```python
from build123d import *

# Parameters (mm, degrees)
CUT_EXTRUDE1_DEPTH             = 115.3
CUT_EXTRUDE1_DEPTH_BACK        = 115.3
BOSS_EXTRUDE1_DEPTH            = 142.875
BOSS_EXTRUDE2_DEPTH            = 22.225
CUT_EXTRUDE2_REACH             = 119.475
CUT_EXTRUDE2_DIRECTION_2_REACH = 119.475


with BuildPart() as part:
    # Sketch1 → Revolve1 (revolve)
    with BuildSketch(Plane(origin=(0, 0, 0), x_dir=(0, 0, -1), z_dir=(1, 0, 0))):
        with BuildLine():
            Line((-76.2, -52.3875), (-117.475, -52.3875))
            Line((-117.475, -52.3875), (-117.475, -114.3))
            Line((-117.475, -114.3), (-95.25, -114.3))
            Line((-95.25, -114.3), (-95.25, -68.2625))
            Line((-95.25, -68.2625), (-76.2, -68.2625))
            Line((-76.2, -68.2625), (-71.4375, -73.025))
            Line((-71.4375, -73.025), (-41.936651857, -73.025))
            ThreePointArc((-41.936651857, -73.025), (-43.560758987, -70.75739219), (-44.836334568, -68.276933343))
            ThreePointArc((-44.836334568, -68.276933343), (-47.073606935, -62.750045829), (-49.120888044, -57.15))
            Line((-49.120888044, -57.15), (-71.4375, -57.15))
            Line((-71.4375, -57.15), (-76.2, -52.3875))
        make_face()
        with BuildLine():
            ThreePointArc((0, -73.025), (15.290494263, -71.406242095), (29.903094423, -66.621734959))
            ThreePointArc((29.903094423, -66.621734959), (31.838045941, -65.273118673), (33.147328418, -63.311338191))
            ThreePointArc((33.147328418, -63.311338191), (34.41368905, -60.243324902), (35.616899689, -57.15))
            Line((35.616899689, -57.15), (49.120888044, -57.15))
            ThreePointArc((49.120888044, -57.15), (47.073606935, -62.750045829), (44.836334568, -68.276933343))
            ThreePointArc((44.836334568, -68.276933343), (40.908487139, -74.162274791), (35.103632583, -78.208123648))
            ThreePointArc((35.103632583, -78.208123648), (17.949710657, -83.824718982), (0, -85.725))
            ThreePointArc((0, -85.725), (-17.949710657, -83.824718982), (-35.103632583, -78.208123648))
            ThreePointArc((-35.103632583, -78.208123648), (-40.908487139, -74.162274791), (-44.836334568, -68.276933343))
            ThreePointArc((-44.836334568, -68.276933343), (-47.073606935, -62.750045829), (-49.120888044, -57.15))
            Line((-49.120888044, -57.15), (-35.616899689, -57.15))
            ThreePointArc((-35.616899689, -57.15), (-34.41368905, -60.243324902), (-33.147328418, -63.311338191))
            ThreePointArc((-33.147328418, -63.311338191), (-31.838045941, -65.273118673), (-29.903094423, -66.621734959))
            ThreePointArc((-29.903094423, -66.621734959), (-15.290494263, -71.406242095), (0, -73.025))
        make_face()
        with BuildLine():
            ThreePointArc((44.836334568, -68.276933343), (43.560758987, -70.75739219), (41.936651857, -73.025))
            Line((41.936651857, -73.025), (71.4375, -73.025))
            Line((71.4375, -73.025), (76.2, -68.2625))
            Line((76.2, -68.2625), (95.25, -68.2625))
            Line((95.25, -68.2625), (95.25, -114.3))
            Line((95.25, -114.3), (117.475, -114.3))
            Line((117.475, -114.3), (117.475, -52.3875))
            Line((117.475, -52.3875), (76.2, -52.3875))
            Line((76.2, -52.3875), (71.4375, -57.15))
            Line((71.4375, -57.15), (49.120888044, -57.15))
            ThreePointArc((49.120888044, -57.15), (47.073606935, -62.750045829), (44.836334568, -68.276933343))
        make_face()
    revolve(axis=Axis((0, 0, 117.475), (0, 0, -1)))

    # Sketch2 → Cut-Extrude1 (cut, two sides)
    with BuildSketch(Plane(origin=(0, 0, 0), x_dir=(0, 0, -1), z_dir=(1, 0, 0))) as cut_extrude1_sk:
        Polygon((-25.4, 0), (-35.399954241, 114.3), (35.399954241, 114.3), (25.4, 0), align=None)
    extrude(amount=CUT_EXTRUDE1_DEPTH, mode=Mode.SUBTRACT)
    extrude(cut_extrude1_sk.sketch, amount=-CUT_EXTRUDE1_DEPTH_BACK, mode=Mode.SUBTRACT)

    # Sketch3 → Boss-Extrude1 (add)
    with BuildSketch(Plane(origin=(0, 142.875, 0), x_dir=(1, 0, 0), z_dir=(0, 1, 0))):
        with BuildLine():
            ThreePointArc((78.208123648, -35.103632583), (85.725, 0), (78.208123648, 35.103632583))
            ThreePointArc((78.208123648, 35.103632583), (74.162274791, 40.908487139), (68.276933343, 44.836334568))
            ThreePointArc((68.276933343, 44.836334568), (0, 58.7375), (-68.276933343, 44.836334568))
            ThreePointArc((-68.276933343, 44.836334568), (-74.162274791, 40.908487139), (-78.208123648, 35.103632583))
            ThreePointArc((-78.208123648, 35.103632583), (-85.725, 0), (-78.208123648, -35.103632583))
            ThreePointArc((-78.208123648, -35.103632583), (-74.162274791, -40.908487139), (-68.276933343, -44.836334568))
            ThreePointArc((-68.276933343, -44.836334568), (0, -58.7375), (68.276933343, -44.836334568))
            ThreePointArc((68.276933343, -44.836334568), (74.162274791, -40.908487139), (78.208123648, -35.103632583))
        make_face()
        with BuildLine():
            ThreePointArc((66.621734959, -29.903094423), (65.273118673, -31.838045941), (63.311338191, -33.147328418))
            ThreePointArc((63.311338191, -33.147328418), (0, -46.0375), (-63.311338191, -33.147328418))
            ThreePointArc((-63.311338191, -33.147328418), (-65.273118673, -31.838045941), (-66.621734959, -29.903094423))
            ThreePointArc((-66.621734959, -29.903094423), (-73.025, 0), (-66.621734959, 29.903094423))
            ThreePointArc((-66.621734959, 29.903094423), (-65.273118673, 31.838045941), (-63.311338191, 33.147328418))
            ThreePointArc((-63.311338191, 33.147328418), (0, 46.0375), (63.311338191, 33.147328418))
            ThreePointArc((63.311338191, 33.147328418), (65.273118673, 31.838045941), (66.621734959, 29.903094423))
            ThreePointArc((66.621734959, 29.903094423), (73.025, 0), (66.621734959, -29.903094423))
        make_face(mode=Mode.SUBTRACT)
    extrude(amount=-BOSS_EXTRUDE1_DEPTH)

    # Sketch3<3> → Boss-Extrude2 (add)
    with BuildSketch(Plane(origin=(0, 142.875, 0), x_dir=(1, 0, 0), z_dir=(0, 1, 0))):
        with BuildLine():
            ThreePointArc((107.174095369, -48.104977984), (117.475, 0), (107.174095369, 48.104977984))
            ThreePointArc((107.174095369, 48.104977984), (96.385165084, 63.584590133), (80.690921224, 74.058849944))
            ThreePointArc((80.690921224, 74.058849944), (0, 90.4875), (-80.690921224, 74.058849944))
            ThreePointArc((-80.690921224, 74.058849944), (-96.385165084, 63.584590133), (-107.174095369, 48.104977984))
            ThreePointArc((-107.174095369, 48.104977984), (-117.475, 0), (-107.174095369, -48.104977984))
            ThreePointArc((-107.174095369, -48.104977984), (-96.385165084, -63.584590133), (-80.690921224, -74.058849944))
            ThreePointArc((-80.690921224, -74.058849944), (0, -90.4875), (80.690921224, -74.058849944))
            ThreePointArc((80.690921224, -74.058849944), (96.385165084, -63.584590133), (107.174095369, -48.104977984))
        make_face()
        with BuildLine():
            ThreePointArc((78.208123648, 35.103632583), (74.162274791, 40.908487139), (68.276933343, 44.836334568))
            ThreePointArc((68.276933343, 44.836334568), (0, 58.7375), (-68.276933343, 44.836334568))
            ThreePointArc((-68.276933343, 44.836334568), (-74.162274791, 40.908487139), (-78.208123648, 35.103632583))
            ThreePointArc((-78.208123648, 35.103632583), (-85.725, 0), (-78.208123648, -35.103632583))
            ThreePointArc((-78.208123648, -35.103632583), (-74.162274791, -40.908487139), (-68.276933343, -44.836334568))
            ThreePointArc((-68.276933343, -44.836334568), (0, -58.7375), (68.276933343, -44.836334568))
            ThreePointArc((68.276933343, -44.836334568), (74.162274791, -40.908487139), (78.208123648, -35.103632583))
            ThreePointArc((78.208123648, -35.103632583), (85.725, 0), (78.208123648, 35.103632583))
        make_face(mode=Mode.SUBTRACT)
    extrude(amount=-BOSS_EXTRUDE2_DEPTH)

    # Sketch5 → Cut-Extrude2 (cut, up to next)
    with BuildSketch(Plane.XY, mode=Mode.PRIVATE) as cut_extrude2_sk1:
        with BuildLine():
            Line((-57.15, 0), (57.15, 0))
            ThreePointArc((57.15, 0), (0, 57.15), (-57.15, 0))
        make_face()
    cut_extrude2_tool1 = extrude(cut_extrude2_sk1.sketch, amount=CUT_EXTRUDE2_REACH, mode=Mode.PRIVATE) & part.part
    add(cut_extrude2_tool1.solids().sort_by_distance((0, 24.255213, 0))[0], mode=Mode.SUBTRACT)

    # Sketch5 → Cut-Extrude2 direction 2 (cut, up to next)
    with BuildSketch(Plane.XY, mode=Mode.PRIVATE) as cut_extrude2_direction_2_sk1:
        with BuildLine():
            Line((-57.15, 0), (57.15, 0))
            ThreePointArc((57.15, 0), (0, 57.15), (-57.15, 0))
        make_face()
    cut_extrude2_direction_2_tool1 = extrude(cut_extrude2_direction_2_sk1.sketch, amount=-CUT_EXTRUDE2_DIRECTION_2_REACH, mode=Mode.PRIVATE) & part.part
    add(cut_extrude2_direction_2_tool1.solids().sort_by_distance((0, 24.255213, 0))[0], mode=Mode.SUBTRACT)


solid = part.part
```
Could you check a few things on this model? Use its own coordinates, in mm. A direction names the side the tool comes from. Round coordinates to 2 decimals unless told otherwise and drop trailing zeros. Loops run counter-clockwise (first coordinate to the right, second up) from the corner with the lowest first, then second, coordinate; pieces in that order, holes last. Notation, with made-up numbers: (-32.75, 12.25) - (-25.75, 12.25) arc R10 ccw to (-25.75, 28.25) - close; hole circle Ø2 at (-21.75, 52.25). An arc over 180 degrees is marked (long way). Answer in a Markdown table with one row per item. Add a question column.
(1) If we section it at A-A (x = 101): Please give me the cut outline in (y, z) (3 decimals), plus the area to 3 significant figures.
(2) I'm going to push flat-ended pins straight in: pin 1 (3 mm diameter, centred on x = 18.5, z = 43.5, fed in from -Y); pin 2 (3 mm diameter, centred on y = -0.5, z = 9, fed in from -X); pin 3 (10 mm diameter, centred on x = -31.5, z = -31, fed in from -Y). Where does each tip first touch, or does it pass through?
(3) If we mould it in two halves opening along Z, with no side actions, what happens to faces 6 (the face through (-15.805, -50.189, 75.969)), 7 (the face through (96.195, 131.918, 63.77)), 8 (the face through (-5.03, 114.19, 106.21)), 9 (the face through (-96.195, 131.918, -63.77))? For each: pulls with the +Z half, pulls with the -Z half, needs draft (parallel to the pull), parting line crosses it, or undercut.
(4) For faces 1 (the face through (74.09, 61.17, 40.98)), 2 (the face through (-74.23, 61.17, 40.84)), 3 (the face through (1.161, 131.918, -90.484)), 4 (the face through (-4.75, 65.97, 31.17)), 5 (the face through (51.433, 11.421, -75.902)), which set-ups out of +Z, -Z, +X, -X, +Y, -Y let a thin tool reach every point of the face, with its end or its side?
(5) If we section it at B-B (z = 13.5): Please give me the cut outline in (x, y) (3 decimals), plus the area to 3 significant figures.
(6) If we section it at C-C (x = 0): State how many separate pieces and enclosed holes the cut face has, plus the area to 3 significant figures.
(7) I need wall thicknesses on line 1 along Y through (x, z) = (0, 60) (3 decimals); line 2 along X through (y, z) = (0, 48) (3 decimals); line 3 along Z through (x, y) = (98, 31.5) (3 decimals). Which ranges of each line are inside material? Lowest first, please.
Model answer:
| question | item | result |
|---|---|---|
| 1 | outline | (-53.512, -117.475) - (53.512, -117.475) - (53.512, -95.25) - (-53.512, -95.25) - close; (-53.512, 95.25) - (53.512, 95.25) - (53.512, 117.475) - (-53.512, 117.475) - close; (120.65, -58.398) - (142.875, -58.398) - (142.875, 58.398) - (120.65, 58.398) - close |
| 1 | area | 7,350 mm² |
| 2 | pin 1 | stops at y = -71.02 |
| 2 | pin 2 | stops at x = -85.4 |
| 2 | pin 3 | stops at y = -76.24 |
| 3 | face 6 | undercut |
| 3 | face 7 | pulls with the +Z half |
| 3 | face 8 | needs draft |
| 3 | face 9 | pulls with the -Z half |
| 4 | face 1 | +X |
| 4 | face 2 | -X |
| 4 | face 3 | -Z, +Y |
| 4 | face 4 | +Y |
| 4 | face 5 | none |
| 5 | outline | (-116.697, 120.65) - (-84.655, 120.65) - (-84.655, 0) arc R84.655 ccw to (84.655, 0) - (84.655, 120.65) - (116.697, 120.65) - (116.697, 142.875) - (71.766, 142.875) - (71.766, 0) arc R71.766 cw to (-71.766, 0) - (-71.766, 142.875) - (-116.697, 142.875) - close |
| 5 | area | 8,270 mm² |
| 6 | separate pieces | 3 |
| 6 | enclosed holes | 0 |
| 6 | area | 13,600 mm² |
| 7 | line 1 | y = -73.025 to -57.15, 57.15 to 73.025, 120.65 to 142.875 |
| 7 | line 2 | x = -73.025 to -57.15, 57.15 to 73.025 |
| 7 | line 3 | z = -117.475 to -95.25, 95.25 to 117.475 |
